```python
from build123d import *

# Parameters (mm, degrees)
SKETCH1_R           = 1.75
BOSS_EXTRUDE1_DEPTH = 2.7


with BuildPart() as part:
    # Sketch1 → Boss-Extrude1 (new body)
    with BuildSketch(Plane.XY):
        with BuildLine():
            Line((142.5, 205.819306835), (141, 205.819306835))
            ThreePointArc((141, 205.819306835), (140.292893219, 206.112200054), (140, 206.819306835))
            Line((140, 206.819306835), (140, 217.457909006))
            ThreePointArc((140, 217.457909006), (139.707106781, 218.165015787), (139, 218.457909006))
            Line((139, 218.457909006), (121.5, 218.457909006))
            ThreePointArc((121.5, 218.457909006), (120.792893219, 218.165015787), (120.5, 217.457909006))
            Line((120.5, 217.457909006), (120.5, 104.457909006))
            ThreePointArc((120.5, 104.457909006), (120.792893219, 103.750802225), (121.5, 103.457909006))
            Line((121.5, 103.457909006), (142.5, 103.457909006))
            ThreePointArc((142.5, 103.457909006), (143.207106781, 103.750802225), (143.5, 104.457909006))
            Line((143.5, 104.457909006), (143.5, 204.819306835))
            ThreePointArc((143.5, 204.819306835), (143.207106781, 205.526413617), (142.5, 205.819306835))
        make_face()
        with Locations(Location((130, 200.941258447, 0), (0, 0, 180))):
            Circle(SKETCH1_R, mode=Mode.SUBTRACT)
        with Locations(Location((130, 120.941258447, 0), (0, 0, 180))):
            Circle(SKETCH1_R, mode=Mode.SUBTRACT)
    extrude(amount=BOSS_EXTRUDE1_DEPTH)


solid = part.part
```
Source: CAD feature listing. Evaluate the final solid. Frame: model axes, mm. A direction names the side the tool comes from. Give positions to 0.01 mm unless a question says otherwise; leave off trailing zeros. Write each loop counter-clockwise with the first axis right and the second up, starting at its lowest first coordinate (ties: lowest second). Pieces come first, ordered by that corner, then holes.
1. Access query for faces 1 (the face through (140, 212, 1)), 2 (the face through (132, 162, 2.7)). Directions: +Z, -Z, +X, -X, +Y, -Y. A direction counts if a zero-diameter tool reaches every point of the face in a straight line with its end or side. Return the directions, or none.
2. Material intervals for line 1 along Y through (x, z) = (130, 0.8); line 2 along Y through (x, z) = (131.5, 2.3); line 3 along X through (y, z) = (211, 0.6), sorted ascending.
3. Section query B-B (z = 1.5). Return the cut outline in (x, y).
4. First-contact query: pin 1 (4.5 mm diameter, centred on x = 130, y = 120.94, fed in from +Z); pin 2 (1.2 mm diameter, centred on x = 141.5, z = 1.5, fed in from +Y). Flat tips, straight axial feed; report the tip coordinate or a pass-through.
5. Pull-direction query (Y, two-part tool) for faces 3 (the face through (128.383, 121.612, 1.331)), 4 (the face through (132, 103.458, 1)), 5 (the face through (130, 218.458, 1)), 6 (the face through (128.33, 200.42, 1.33)); classes: +Y half, -Y half, draft (parallel to the pull), parting line (faces both ways), or undercut.
6. Section query A-A (x = 130). Return the cut outline in (y, z).
Output values:
1. face 1: +Z, -Z, +X, +Y
1. face 2: +Z, +X, -X, +Y, -Y
2. line 1: y = 103.46 to 119.19, 122.69 to 199.19, 202.69 to 218.46
2. line 2: y = 103.46 to 120.04, 121.84 to 200.04, 201.84 to 218.46
2. line 3: x = 120.5 to 140
3. outline: (120.5, 104.46) arc R1 ccw to (121.5, 103.46) - (142.5, 103.46) arc R1 ccw to (143.5, 104.46) - (143.5, 204.82) arc R1 ccw to (142.5, 205.82) - (141, 205.82) arc R1 cw to (140, 206.82) - (140, 217.46) arc R1 ccw to (139, 218.46) - (121.5, 218.46) arc R1 ccw to (120.5, 217.46) - close; hole circle Ø3.5 at (130, 120.94); hole circle Ø3.5 at (130, 200.94)
4. pin 1: stops at z = 2.7
4. pin 2: stops at y = 205.82
5. face 3: undercut
5. face 4: -Y half
5. face 5: +Y half
5. face 6: undercut
6. outline: (103.46, 0) - (119.19, 0) - (119.19, 2.7) - (103.46, 2.7) - close; (122.69, 0) - (199.19, 0) - (199.19, 2.7) - (122.69, 2.7) - close; (202.69, 0) - (218.46, 0) - (218.46, 2.7) - (202.69, 2.7) - close
